The model under review builds one solid part; all positions refer to its coordinate system, in mm. Face numbers are marked on the shaded views. Coordinates: 2 decimals unless noted, no trailing zeros. Loops run counter-clockwise (first coordinate to the right, second up) from the corner with the lowest first, then second, coordinate; pieces in that order, holes last. Notation, with made-up numbers: M 56.5,24 L 67.5,24 A29 cw 67.5,57 Z; hole C 81,-34 d4. An arc over 180 degrees is marked long. Use CSV: the item, a comma, the result in double quotes. Start each with the question number.
1. Add section B-B, the plane y = 0. Write out the cut boundary in (x, z).
2. Add section A-A, the plane x = -5. Write out the cut boundary in (y, z).
3. Clearance check with flat-ended pins moving along their axes: P1, Ø3, axis at x = 5, y = 1, coming from the -Z side; P2, Ø2.5, axis at x = 5, y = 0, coming from the -Z side. State where each tip first meets the part, or that it passes through.
4. For L1, parallel to X at y = 0, z = 8.65; L2, parallel to Y at x = 5, z = 2.75; L3, parallel to Y at x = 5, z = 8.9, list the stretches that pass through material, from the lowest coordinate up.
5. Add section C-C, the plane z = 9.25. Write out the cut boundary in (x, y).
6. Add section D-D, the plane z = 6.75. Write out the cut boundary in (x, y), then the cut area to 3 significant figures.
7. Draft analysis for pull direction X (two halves, no side actions). For the marked faces 1, 2, 3 and 4, state which applies: +X half, -X half, draft (parallel to the pull), parting line (faces both ways), or undercut.
from build123d import *

# Parameters (mm, degrees)
SKETCH1_W           = 20
SKETCH1_H           = 9
BOSS_EXTRUDE1_DEPTH = 20
SKETCH1_10_R        = 2
CUT_EXTRUDE2_DEPTH  = 10
SKETCH2_R           = 2.75
CUT_EXTRUDE1_DEPTH  = 7


with BuildPart() as part:
    # Sketch1 → Boss-Extrude1 (new body)
    with BuildSketch(Plane.XY):
        with Locations((0, -0.5)):
            Rectangle(SKETCH1_W, SKETCH1_H)
    extrude(amount=BOSS_EXTRUDE1_DEPTH)

    # Sketch1<10> → Cut-Extrude2 (cut)
    with BuildSketch(Plane.XY):
        with Locations((-5, 0)):
            Circle(SKETCH1_10_R)
        with Locations((5, 0)):
            Circle(SKETCH1_10_R)
    extrude(amount=CUT_EXTRUDE2_DEPTH, mode=Mode.SUBTRACT)

    # Sketch2 → Cut-Extrude1 (cut)
    with BuildSketch(Plane.XY):
        with Locations((-5, 0)):
            Circle(SKETCH2_R)
        with Locations((5, 0)):
            Circle(SKETCH2_R)
    extrude(amount=CUT_EXTRUDE1_DEPTH, mode=Mode.SUBTRACT)


solid = part.part
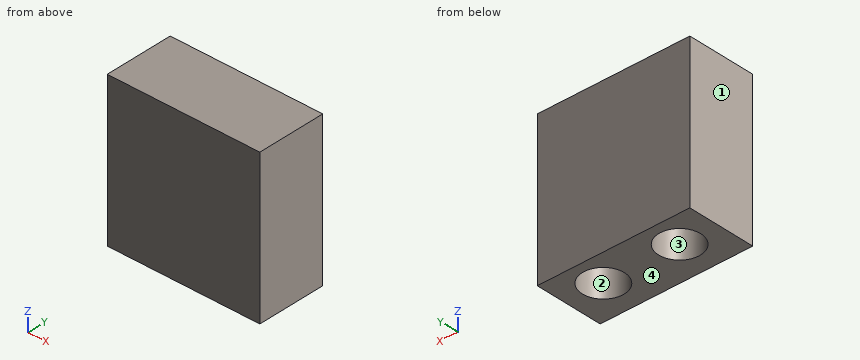
Computed:
1,outline,"M -10,0 L -7.75,0 L -7.75,7 L -7,7 L -7,10 L -3,10 L -3,7 L -2.25,7 L -2.25,0 L 2.25,0 L 2.25,7 L 3,7 L 3,10 L 7,10 L 7,7 L 7.75,7 L 7.75,0 L 10,0 L 10,20 L -10,20 Z"
2,outline,"M -5,0 L -2.75,0 L -2.75,7 L -2,7 L -2,10 L 2,10 L 2,7 L 2.75,7 L 2.75,0 L 4,0 L 4,20 L -5,20 Z"
3,P1,"stops at z = 7"
3,P2,"stops at z = 10"
4,L1,"x = -10 to -7, -3 to 3, 7 to 10"
4,L2,"y = -5 to -2.75, 2.75 to 4"
4,L3,"y = -5 to -2, 2 to 4"
5,outline,"M -10,-5 L 10,-5 L 10,4 L -10,4 Z; hole C -5,0 d4; hole C 5,0 d4"
6,outline,"M -10,-5 L 10,-5 L 10,4 L -10,4 Z; hole C -5,0 d5.5; hole C 5,0 d5.5"
6,area,"132 mm^2"
7,face 1,"-X half"
7,face 2,"undercut"
7,face 3,"undercut"
7,face 4,"draft"
